CAD build for the part. Positions are in the model's coordinates, mm. A direction names the side the tool comes from. Coordinates: 2 decimals unless noted, no trailing zeros. Loops run counter-clockwise (first coordinate to the right, second up) from the corner with the lowest first, then second, coordinate; pieces in that order, holes last.
1) Saw through at B-B, the plane x = -0.7. Write the cut outline in (y, z), and give its area (3 significant figures).
2) Which spindle directions (+Z, -Z, +X, -X, +Y, -Y) get a long thin tool onto all of the face, cutting with end or side? Do faces 1 (the cylindrical face through (-8, 6, 0)), 2 (the flat face through (-15, 0.4, 0)). Say none if no direction does.
3) Saw through at C-C, the plane y = 3. Write the cut outline in (x, z), and give its area (3 significant figures).
4) Two-plate mould, pull along Z, no slides. Class faces 3 (the flat face through (-1, 0.4, 0)), 4 (the cylindrical face through (-15.796, 0.197, 2.935)), 5 (the flat face through (-9.2, 6.1, -5)), 6 (the flat face through (-9.2, 6.1, 5)): +Z half, -Z half, draft (parallel to the pull), parting line (faces both ways), or undercut.
5) Pin check, flat tips, straight feed: pin 1 Ø0.5 at (x, z) = (-1, 0.5) entering from +Y; pin 2 Ø2 at (y, z) = (3, 0.5) entering from -X; pin 3 Ø1.5 at (x, y) = (-14.5, 5.5) entering from -Z; pin 4 Ø1 at (x, z) = (-5.5, 3.5) entering from +Y. Stop position of each tip, or through.
6) Wall check: line 1 along Z through (x, y) = (-15.3, 0.3); line 2 along X through (y, z) = (0.2, 3); line 3 along X through (y, z) = (2.5, -2.75). Give the ranges that are in metal, low to high.
Autodesk Inventor part; units mm, degrees
ref_plane "YZ Plane" through (0, 0, 0) normal (1, 0, 0) x (0, 1, 0)
ref_plane "XZ Plane" through (0, 0, 0) normal (0, 1, 0) x (-1, 0, 0)
ref_plane "XY Plane" through (0, 0, 0) normal (0, 0, 1) x (1, 0, 0)
sketch "Esboço1" plane through (0, 0, 0) normal (0, 0, 1) x (1, 0, 0)
  line L0 (0, 0) -> (-2, 0)
  arc A0 (-2, 0) -> (-14, 0) centre (-8, 0) ccw
  line L1 (-14, 0) -> (-16, 0)
  line L2 (-16, 0.4) -> (-14.3875, 0.4)
  arc A1 (-1.6125, 0.4) -> (-14.3875, 0.4) centre (-8, 0) ccw
  line L3 (-1.6125, 0.4) -> (0, 0.4)
  line L4 (0, 0.4) -> (0, 0)
  line L5 (-16, 0.4) -> (-16, 0)
  dimension "d2" = 2
  dimension "d3" = 12
  dimension "d4" = 6
  dimension "d5" = 2
  dimension "d6" = 6.4
extrude "Extrusão1" add sketch "Esboço1" along normal mid plane 10
sketch "Esboço4" plane through (-1.6125, 0.4, 5) normal (0, 1, 0) x (1, 0, 0)
  line L0 (1.6125, 10) -> (1.6125, 0)
  line L1 (1.6125, 0) -> (0, 0)
  line L2 (0, 10) -> (1.6125, 10)
  point P0 (1.6125, 5)
  point P1 (0.9125, 2)
  point P2 (0.9125, 8)
  point P3 (0.8063, 0)
  dimension "d13" = 0.7
  dimension "d14" = 0.7
  dimension "d15" = 2
  dimension "d16" = 2
hole "Furo1" at (-0.7, 0.4, 3) at (-0.7, 0.4, -3) direction (0, -1, 0) diameter 0.5 end through all counterbore diameter 1 counterbore depth 1
sketch "Esboço5" plane through (-16, 0.4, 5) normal (0, 1, 0) x (1, 0, 0)
  line L0 (0, 10) -> (0, 0)
  line L1 (0, 10) -> (1.6125, 10)
  line L2 (1.6125, 0) -> (0, 0)
  point P0 (16, 5)
  point P1 (0.7, 8)
  point P2 (0.7, 2)
  dimension "d24" = 0.7
  dimension "d25" = 2
  dimension "d26" = 2
  dimension "d27" = 0.7
hole "Furo2" at (-15.3, 0.4, -3) at (-15.3, 0.4, 3) direction (0, -1, 0) diameter 0.5 end through all counterbore diameter 1 counterbore depth 1
thread "Rosca1"
thread "Rosca2"
thread "Rosca3"
thread "Rosca4"
thread "Rosca5"
equation "\"Raio_vergadura\" = Espessura"
equation "\"Largura_alívio_de_vergadura\" = Espessura"
equation "\"Profundidade_alívio_de_vergadura\" = 0.5 * Espessura"
equation "\"Tamanho_alívio_de_dobra\" = 4 * Espessura"
equation "\"Remanescente_mínimo\" = 2 * Espessura"
equation "\"Raiodetransição\" = Raio_vergadura"
equation "\"Tamanho_de_raio_de_Jacobi\" = Raio_vergadura"
equation "\"TamanhoFolga\" = Espessura"
Data:
1. outline: (0, -5) - (0.4, -5) - (0.4, -3.5) - (0, -3.5) - close; (0, -2.5) - (0.4, -2.5) - (0.4, 2.5) - (0, 2.5) - close; (0, 3.5) - (0.4, 3.5) - (0.4, 5) - (0, 5) - close
1. area: 3.20 mm2
2. face 1: +Z, -Z, -Y
2. face 2: +Z, -Z, -X, +Y
3. outline: (-13.65, -5) - (-13.2, -5) - (-13.2, 5) - (-13.65, 5) - close; (-2.8, -5) - (-2.35, -5) - (-2.35, 5) - (-2.8, 5) - close
3. area: 9.14 mm2
4. face 3: draft
4. face 4: undercut
4. face 5: -Z half
4. face 6: +Z half
5. pin 1: stops at y = 0.4
5. pin 2: stops at x = -14.08
5. pin 3: passes through
5. pin 4: stops at y = 6.08
6. line 1: z = -5 to -3.5, -2.5 to 2.5, 3.5 to 5
6. line 2: x = -16 to -15.8, -14.8 to -14, -2 to -1.2, -0.2 to 0
6. line 3: x = -13.89 to -13.45, -2.55 to -2.11
